Work out the finished part from the listing and answer in its coordinate system (mm). Give positions to 0.01 mm unless a question says otherwise; leave off trailing zeros. Order: outer loops, then holes, each group sorted by start corner. A loop starts at its lowest first (then second) coordinate and runs counter-clockwise, first axis right, second up.
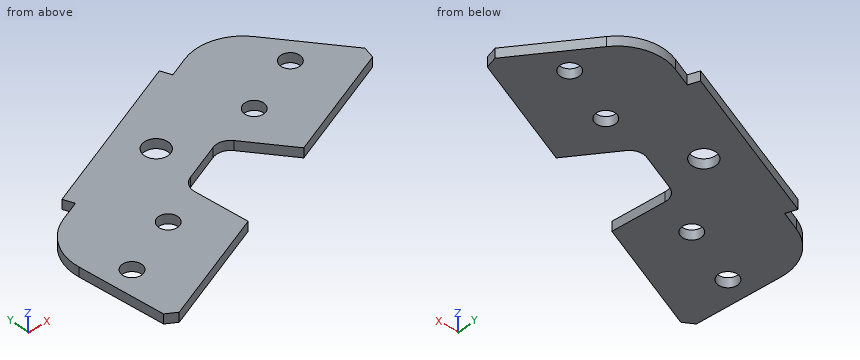
```python
from build123d import *

# Parameters (mm, degrees)
SKETCH_1_W          = 178.1038796
SKETCH_1_H          = 112.631890056
EXTRUDE_1_DEPTH     = 2
SKETCH_2_OUTSIDE_W  = 222.252
SKETCH_2_OUTSIDE_H  = 156.78
CUT_EXTRUDE_1_DEPTH = 2
SKETCH_3_R          = 2
CUT_EXTRUDE_2_DEPTH = 2
SKETCH_4_R          = 2
CUT_EXTRUDE_3_DEPTH = 10
SKETCH_5_R          = 2.5
CUT_EXTRUDE_4_DEPTH = 10


with BuildPart() as part:
    # 草图1 → 凸台-拉伸1 (new body)
    with BuildSketch(Plane.XY):
        Rectangle(SKETCH_1_W, SKETCH_1_H)
    extrude(amount=EXTRUDE_1_DEPTH)

    # 草图2 outside → 切除-拉伸1 (cut)
    with BuildSketch(Plane.XY.offset(2)):
        Rectangle(SKETCH_2_OUTSIDE_W, SKETCH_2_OUTSIDE_H)
        with BuildLine():
            Line((19.419678114, -9.00835621), (26.240314518, -17.576109786))
            Line((26.240314518, -17.576109786), (49.120442624, -8.088240876))
            Line((49.120442624, -8.088240876), (49.672051155, -5.694361888))
            Line((49.672051155, -5.694361888), (38.815198664, 7.943491127))
            ThreePointArc((38.815198664, 7.943491127), (33.491549784, 11.397714714), (27.161091097, 10.952528456))
            Line((27.161091097, 10.952528456), (23.209000469, 9.31368633))
            Line((23.209000469, 9.31368633), (22.32798775, 11.438260779))
            Line((22.32798775, 11.438260779), (-10.002492997, -1.968454504))
            Line((-10.002492997, -1.968454504), (-9.121480278, -4.093028953))
            Line((-9.121480278, -4.093028953), (-13.073570906, -5.731871079))
            ThreePointArc((-13.073570906, -5.731871079), (-17.86138023, -9.897177774), (-19.178350627, -16.105115191))
            Line((-19.178350627, -16.105115191), (-17.198178577, -33.42392576))
            Line((-17.198178577, -33.42392576), (-15.114374014, -34.724958857))
            Line((-15.114374014, -34.724958857), (7.765754091, -25.237089947))
            Line((7.765754091, -25.237089947), (6.521744045, -14.356836213))
            ThreePointArc((6.521744045, -14.356836213), (6.916835164, -12.494454989), (8.353177961, -11.24486298))
            Line((8.353177961, -11.24486298), (15.923445844, -8.105645011))
            ThreePointArc((15.923445844, -8.105645011), (17.82258345, -7.972089134), (19.419678114, -9.00835621))
        make_face(mode=Mode.SUBTRACT)
    extrude(amount=-CUT_EXTRUDE_1_DEPTH, mode=Mode.SUBTRACT)

    # 草图3 → 切除-拉伸2 (cut)
    with BuildSketch(Plane.XY.offset(2)):
        with Locations((39.039313187, -0.266244108)):
            Circle(SKETCH_3_R)
        with Locations((-13.526945878, -22.064276566)):
            Circle(SKETCH_3_R)
    extrude(amount=-CUT_EXTRUDE_2_DEPTH, mode=Mode.SUBTRACT)

    # 草图4 → 切除-拉伸3 (cut)
    with BuildSketch(Plane.XY.offset(2)):
        with Locations((-1.5184816, -17.084639461)):
            Circle(SKETCH_4_R)
        with Locations((27.030848909, -5.245881212)):
            Circle(SKETCH_4_R)
    extrude(amount=-CUT_EXTRUDE_3_DEPTH, mode=Mode.SUBTRACT)

    # 草图5 → 切除-拉伸4 (cut)
    with BuildSketch(Plane.XY.offset(2)):
        with Locations((9.15052964, -2.470175429)):
            Circle(SKETCH_5_R)
    extrude(amount=-CUT_EXTRUDE_4_DEPTH, mode=Mode.SUBTRACT)


solid = part.part
```
1. The part is cut by section C-C (x = 43). Write down the section's boundary in (y, z).
Findings below:
outline: (-10.63, 0) - (2.69, 0) - (2.69, 2) - (-10.63, 2) - close
2. Straight lines are drawn through the part: probe 1 along X at (y, z) = (-4.5, 0.95); probe 2 along X at (y, z) = (-16, 0.5); probe 3 along Y at (x, z) = (10, 0.25). For each, find the intervals that lie inside material, in ascending order.
Findings below:
probe 1: x = -10.1 to 7.69, 10.61 to 25.18, 28.89 to 48.72
probe 2: x = -19.19 to -3.2, 0.16 to 6.71, 24.99 to 30.04
probe 3: y = -10.56 to -4.82, -0.12 to 6.33
3. The part is cut by section D-D (y = -30). Write down the section's boundary in (x, z).
Findings below:
outline: (-17.59, 0) - (-3.72, 0) - (-3.72, 2) - (-17.59, 2) - close
4. The part is cut by section A-A (z = 1.15). Write down the section's boundary in (x, y).
Findings below:
outline: (-19.18, -16.11) - (-17.2, -33.42) - (-15.11, -34.72) - (7.77, -25.24) - (6.52, -14.36) arc R3 cw to (8.35, -11.24) - (15.92, -8.11) arc R3 cw to (19.42, -9.01) - (26.24, -17.58) - (49.12, -8.09) - (49.67, -5.69) - (38.82, 7.94) arc R10 ccw to (27.16, 10.95) - (23.21, 9.31) - (22.33, 11.44) - (-10, -1.97) - (-9.12, -4.09) - (-13.07, -5.73) arc R10 ccw to start; hole circle Ø4 at (-13.53, -22.06); hole circle Ø4 at (-1.52, -17.08); hole circle Ø5 at (9.15, -2.47); hole circle Ø4 at (27.03, -5.25); hole circle Ø4 at (39.04, -0.27)
5. The part is cut by section B-B (y = -10.5). Write down the section's boundary in (x, z).
Findings below:
outline: (-18.19, 0) - (10.15, 0) - (10.15, 2) - (-18.19, 2) - close; (20.61, 0) - (43.3, 0) - (43.3, 2) - (20.61, 2) - close
